Autodesk Inventor part; units mm, degrees
ref_plane "YZ Plane" through (0, 0, 0) normal (1, 0, 0) x (0, 1, 0)
ref_plane "XZ Plane" through (0, 0, 0) normal (0, 1, 0) x (-1, 0, 0)
ref_plane "XY Plane" through (0, 0, 0) normal (0, 0, 1) x (1, 0, 0)
sketch "Esboço1" plane through (0, 0, 0) normal (0, 0, 1) x (1, 0, 0)
  arc A0 (-10, 0) -> (10, 0) centre (0, 0) ccw
  line L0 (10, 0) -> (90, 0)
  line L1 (90, 0) -> (90, 10)
  line L2 (90, 10) -> (-65, 10)
  line L3 (-65, 10) -> (-65, -5)
  line L4 (-65, -5) -> (-50, -5)
  line L5 (-50, -5) -> (-41.3397, 0)
  line L6 (-41.3397, 0) -> (-10, 0)
  dimension "d0" = 20
  dimension "d1" = 155
  dimension "d2" = 90
  dimension "d3" = 15
  dimension "d4" = 30
  dimension "d5" = 10
  dimension "d6" = 15
extrude "Extrusão1" add sketch "Esboço1" along normal mid plane 12
fillet "Arredondamento1" radius 5 1 edges at (-65, 10, 0)
sketch "Esboço2" plane through (0, 0, 6) normal (0, 0, 1) x (1, 0, 0)
  circle A0 centre (0, 0) radius 5
  dimension "d10" = 10
extrude "Extrusão2" cut sketch "Esboço2" against normal through all
sketch "Esboço3" plane through (90, 10, 6) normal (0, 1, 0) x (1, 0, 0)
  circle A0 centre (-10, 6) radius 10
  line L0 (0, 12) -> (0, 0)
  line L1 (-150, 0) -> (-150, 12)
  point P0 (-90, 6)
  point P1 (-150, 6)
  dimension "d13" = 20
  dimension "d14" = 10
extrude "Extrusão3" add sketch "Esboço3" against normal blind 10
properties material "Liga de aço"
The model under review builds one solid part; all positions refer to its coordinate system, in mm. A direction names the side the tool comes from. Give positions to 0.01 mm unless a question says otherwise; leave off trailing zeros. Write each loop counter-clockwise with the first axis right and the second up, starting at its lowest first coordinate (ties: lowest second). Pieces come first, ordered by that corner, then holes. Notation, with made-up numbers: (23, 87) -> (38, 87) arc R15 ccw to (38, 107) -> close; hole circle Ø3 at (-18.75, -38). An arc over 180 degrees is marked (long way). Put each result on its own line as item: value.
(1) We need section A-A, the plane z = -3. Give the boundary of the cut face in (x, y).
Results are:
outline: (-65, -5) -> (-50, -5) -> (-41.34, 0) -> (-10, 0) arc R10 ccw to (10, 0) -> (90, 0) -> (90, 10) -> (-60, 10) arc R5 ccw to (-65, 5) -> close; hole circle Ø10 at (0, 0)
(2) Tool access review of faces 4 (the flat face through (-45.73, -2.535, -0.084)), 5 (the flat face through (3, 5, 6)), 6 (the flat face through (-58, -5, 0)): name each direction out of +Z, -Z, +X, -X, +Y, -Y from which nothing blocks a thin tool from reaching the whole face with its end or side.
Results are:
face 4: +Z, -Z, -Y
face 5: +Z, -X, +Y, -Y
face 6: +Z, -Z, -X, -Y
(3) For pin 1 Ø9.5 at (x, z) = (-59.5, -1) entering from -Y; pin 2 Ø2 at (y, z) = (-7, 0.5) entering from -X, all flat-tipped, find the tip position at first contact; note any pin that passes through.
Results are:
pin 1: y = -5
pin 2: x = -8
(4) The part is to be moulded in two halves that separate along Y. For faces 1 (the cylindrical face through (80, 5, 10)), 2 (the cylindrical face through (-1.08, -4.88, 0.08)), 3 (the flat face through (49, 0, 0)), say which applies: pulls with the +Y half, pulls with the -Y half, needs draft (parallel to the pull), parting line crosses it, or undercut.
Results are:
face 1: needs draft
face 2: undercut
face 3: pulls with the -Y half
(5) We need section B-B, the plane x = 0. Give the boundary of the cut face in (y, z), and give its area (3 significant figures).
Results are:
outline: (-10, -6) -> (-5, -6) -> (-5, 6) -> (-10, 6) -> close; (5, -6) -> (10, -6) -> (10, 6) -> (5, 6) -> close
area: 120 mm²
(6) We need section D-D, the plane x = 33. Give the boundary of the cut face in (y, z).
Results are:
outline: (0, -6) -> (10, -6) -> (10, 6) -> (0, 6) -> close
(7) To check wall thickness, follow probe 1 along Y at (x, z) = (0, -2.75); probe 2 along Y at (x, z) = (-34.5, 3.75); probe 3 along Z at (x, y) = (-20.5, 8). State the ranges of each line that lie inside material, in increasing order. Write a range as from..to.
Results are:
probe 1: -10..-5, 5..10
probe 2: 0..10
probe 3: -6..6
(8) We need section C-C, the plane y = 2.25. Give the boundary of the cut face in (x, z), and give its area (3 significant figures).
Results are:
outline: (-65, -6) -> (-4.47, -6) -> (-4.47, 6) -> (-65, 6) -> close; (4.47, -6) -> (72, -6) arc R10 ccw to (88, -6) -> (90, -6) -> (90, 6) -> (88, 6) arc R10 ccw to (72, 6) -> (4.47, 6) -> close
area: 1,840 mm²
